Autodesk Inventor part; units mm, degrees
ref_plane "YZ Plane" through (0, 0, 0) normal (1, 0, 0) x (0, 1, 0)
ref_plane "XZ Plane" through (0, 0, 0) normal (0, 1, 0) x (-1, 0, 0)
ref_plane "XY Plane" through (0, 0, 0) normal (0, 0, 1) x (1, 0, 0)
sketch "Sketch1" plane through (0, 0, 0) normal (0, 1, 0) x (-1, 0, 0)
  circle A0 centre (0, 0) radius 4
  dimension "d0" = 8
extrude "Extrusion1" add sketch "Sketch1" along normal blind 5
sketch "Sketch2" plane through (0, 5, 0) normal (0, 1, 0) x (1, 0, 0)
  circle A0 centre (0, 0) radius 2.5
  dimension "d3" = 5
extrude "Extrusion2" add sketch "Sketch2" along normal blind 40
sketch "Sketch3" plane through (0, 0, 0) normal (0, -1, 0) x (1, 0, 0)
  line L0 (2.8865, -0.0416) -> (1.4072, -2.5205)
  line L1 (1.4072, -2.5205) -> (-1.4792, -2.479)
  line L2 (-1.4792, -2.479) -> (-2.8865, 0.0416)
  line L3 (-2.8865, 0.0416) -> (-1.4072, 2.5205)
  line L4 (-1.4072, 2.5205) -> (1.4792, 2.479)
  line L5 (1.4792, 2.479) -> (2.8865, -0.0416)
  point P0 (0, 0)
  point P1 (0, 0)
  dimension "d6" = 2.5
extrude "Extrusion3" cut sketch "Sketch3" against normal blind 3
fillet "Fillet1" radius 0.5 1 edges at (4, 0, 0)
fillet "Fillet2" radius 0.5 2 edges at (-2.5, 5, 0) (-2.5, 45, 0)
properties part number "bulong5mmdai50"
Verification items for the finished model (mm, model axes). A direction names the side the tool comes from. Give positions to 0.01 mm unless a question says otherwise; leave off trailing zeros. Order: outer loops, then holes, each group sorted by start corner. A loop starts at its lowest first (then second) coordinate and runs counter-clockwise, first axis right, second up. Notation, with made-up numbers: M -7,-8.75 L -1,-8.75 A19 ccw -1,13.25 Z; hole C 14.25,28 d9. An arc over 180 degrees is marked long. Answer in a Markdown table with one row per item. Add a question column.
Item 1: Section check B-B, the plane x = 0. Enter the section's corners in (y, z).
Item 2: Tool access check on faces 5 (the flat face through (-1, 5, 3)), 6 (the flat face through (-2.17, 1.48, -1.24)), 7 (the flat face through (2, 0, -2)). Record the directions out of +Z, -Z, +X, -X, +Y, -Y that give a thin tool (end or side, any length) a straight path to the whole face; none if there is none.
Item 3: Mould release check, pull along Z, two halves, no side actions. Record for faces 1 (the flat face through (-2.16, 1.48, 1.26)), 2 (the flat face through (0, 45, 0)), 3 (the cylindrical face through (0.867, 2.718, 3.905)), 4 (the flat face through (0, 3, 0)): released by +Z, released by -Z, zero draft, split by the parting line, or undercut.
Item 4: Gauge pin test, flat end, axial feed: pin 1 (2 mm diameter, centred on y = 39, z = -1.5, fed in from -X). Record the tip position at first contact, or that the pin passes through.
Item 5: Scan lines: probe 1 along Z at (x, y) = (-1.5, 35); probe 2 along Y at (x, z) = (1.25, 3); probe 3 along Z at (x, y) = (0, 17). Record each from-to range of solid material in increasing order. Write a range as from..to.
Item 6: Section check A-A, the plane y = 31. Enter the section's corners in (x, z).
Filled sheet:
| question | item | result |
|---|---|---|
| 1 | outline | M 0,-3.5 A0.5 ccw 0.5,-4 L 5,-4 L 5,-3 A0.5 cw 5.5,-2.5 L 44.5,-2.5 A0.5 ccw 45,-2 L 45,2 A0.5 ccw 44.5,2.5 L 5.5,2.5 A0.5 cw 5,3 L 5,4 L 0.5,4 A0.5 ccw 0,3.5 L 0,2.5 L 3,2.5 L 3,-2.5 L 0,-2.5 Z |
| 2 | face 5 | +Y |
| 2 | face 6 | -Y |
| 2 | face 7 | +Z, -Z, +X, -X, -Y |
| 3 | face 1 | undercut |
| 3 | face 2 | zero draft |
| 3 | face 3 | split by the parting line |
| 3 | face 4 | undercut |
| 4 | pin 1 | stops at x = -2.45 |
| 5 | probe 1 | z = -2..2 |
| 5 | probe 2 | y = 0..5 |
| 5 | probe 3 | z = -2.5..2.5 |
| 6 | outline | C 0,0 d5 |
